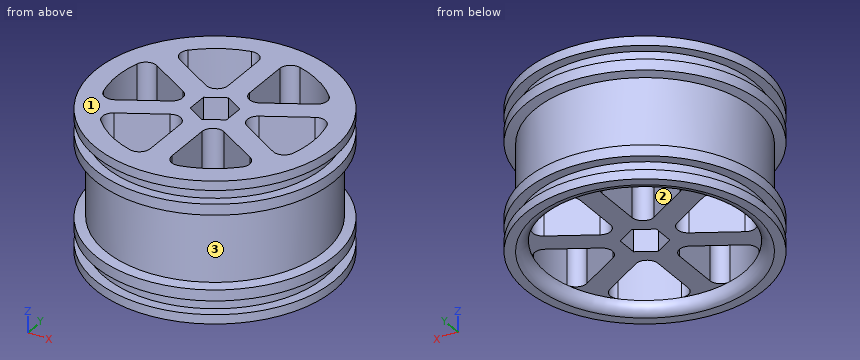
from build123d import *

# Parameters (mm, degrees)
SKETCH2_W               = 4
SKETCH2_H               = 18.2
BOSS_EXTRUDE1_DEPTH     = 24
CIRPATTERN1_COUNT       = 6
CUT_EXTRUDE1_DEPTH      = 41.546269865
CUT_EXTRUDE1_DEPTH_BACK = 41.546269865
FILLET1_R               = 2
FILLET2_R               = 2


with BuildPart() as part:
    # Sketch1 → Revolve1 (revolve)
    with BuildSketch(Plane(origin=(0, 0, 0), x_dir=(0, 0, -1), z_dir=(1, 0, 0)), mode=Mode.PRIVATE) as revolve1_sk:
        Polygon((0, 22), (1.7, 22), (1.7, 20.2), (4.2, 20.2), (4.2, 22), (6.2, 22), (6.5, 20.2), (19.5, 20.2), (19.8, 22), (21.8, 22), (21.8, 20.2), (24.3, 20.2), (24.3, 22), (26, 22), (26, 18.2), (0, 18.2), align=None)
    revolve(revolve1_sk.sketch.rotate(Axis((0, 0, 0.322174052), (0, 0, -1)), 90), axis=Axis((0, 0, 0.322174052), (0, 0, -1)))

    # Sketch2 → Boss-Extrude1 (add)
    with BuildSketch(Plane.XY):
        with Locations((0, 9.1)):
            Rectangle(SKETCH2_W, SKETCH2_H)
    boss_extrude1 = extrude(amount=-BOSS_EXTRUDE1_DEPTH)

    # CirPattern1: Boss-Extrude1 ×6 about axis
    cirpattern1_axis = Axis((0, 0, 0), (0, 0, 1))
    for i in range(1, CIRPATTERN1_COUNT):
        add(boss_extrude1.rotate(cirpattern1_axis, i * 360 / CIRPATTERN1_COUNT))

    # Sketch3 → Cut-Extrude1 (cut, two sides: drawn at the far end of the back side and taken through both)
    with BuildSketch(Plane.XY.offset(-CUT_EXTRUDE1_DEPTH_BACK)):
        Polygon((0, -3.87), (3.351518313, -1.935), (3.351518313, 1.935), (0, 3.87), (-3.351518313, 1.935), (-3.351518313, -1.935), align=None)
    extrude(amount=CUT_EXTRUDE1_DEPTH + CUT_EXTRUDE1_DEPTH_BACK, mode=Mode.SUBTRACT)

    # Fillet1
    fillet1_edges = [part.edges().sort_by_distance(p)[0] for p in [
        (14.666205667, 10.776938867, -12),
        (-14.666205667, 10.776938867, -12),
        (-2, 18.089776118, -12),
        (2, 18.089776118, -12),
        (-16.666205667, 7.312837251, -12),
        (-14.666205667, -10.776938867, -12),
        (-16.666205667, -7.312837251, -12),
        (2, -18.089776118, -12),
        (-2, -18.089776118, -12),
        (14.666205667, -10.776938867, -12),
        (16.666205667, -7.312837251, -12),
        (16.666205667, 7.312837251, -12),
        (4, 0, -12),
        (2, -3.464101615, -12),
        (-2, -3.464101615, -12),
        (-4, 0, -12),
        (2, 3.464101615, -12),
        (-2, 3.464101615, -12),
    ]]
    fillet(fillet1_edges, radius=FILLET1_R)

    # Fillet2
    fillet2_edges = [part.edges().sort_by_distance(p)[0] for p in [
        (-18.2, 0, -26),
    ]]
    fillet(fillet2_edges, radius=FILLET2_R - 0.0001)  # a hair under: the kernel refuses the full size


solid = part.part
Design review of the part built by this model. Coordinates are the model's own, in mm. Face numbers are marked on the shaded views. Round coordinates to 2 decimals unless told otherwise and drop trailing zeros.
Item 1: For pin 1 Ø4.5 at (y, z) = (-13, -10.5) entering from +X; pin 2 Ø4.5 at (y, z) = (-9, -14.5) entering from -X; pin 3 Ø6 at (x, z) = (6, -17.5) entering from +Y, all flat-tipped, find the tip position at first contact; note any pin that passes through.
Item 2: Draft analysis for pull direction Y (two halves, no side actions). For the marked faces 1, 2 and 3, state which applies: released by +Y, released by -Y, zero draft, split by the parting line, or undercut.
Item 3: Wall thickness on L1, parallel to Y at x = 0, z = -8.5; L2, parallel to Y at x = -4, z = -22.5; L3, parallel to Y at x = 0, z = -6: over which ranges is each line inside the solid? List them lowest first.
Item 4: Consider section A-A on y = 0. Count the separate pieces of the cut face and the enclosed holes in it, and give its area (3 significant figures).
Check values:
1. pin 1: stops at x = 17.1
1. pin 2: stops at x = -19.04
1. pin 3: stops at y = 21.62
2. face 1: zero draft
2. face 2: undercut
2. face 3: split by the parting line
3. L1: y = -20.2 to -3.87, 3.87 to 20.2
3. L2: y = -19.8 to -17.7, -4.93 to 4.93, 17.7 to 19.8
3. L3: y = -22 to -3.87, 3.87 to 22
4. separate pieces: 4
4. enclosed holes: 0
4. area: 257 mm2
